Autodesk Inventor part; units mm, degrees
ref_plane "YZ Plane" through (0, 0, 0) normal (1, 0, 0) x (0, 1, 0)
ref_plane "XZ Plane" through (0, 0, 0) normal (0, 1, 0) x (-1, 0, 0)
ref_plane "XY Plane" through (0, 0, 0) normal (0, 0, 1) x (1, 0, 0)
sketch "Sketch1" plane through (0, 0, 0) normal (0, 1, 0) x (-1, 0, 0)
  line L0 (-50, 86.6025) -> (-50, -86.6025)
  line L1 (50, -86.6025) -> (50, 86.6025)
  arc A0 (50, 86.6025) -> (-50, 86.6025) centre (0, 0) ccw
  arc A1 (-50, -86.6025) -> (50, -86.6025) centre (0, 0) ccw
  circle A2 centre (42, -84.8528) radius 1.3
  circle A3 centre (42, -60.6528) radius 1.3
  circle A4 centre (-42, -84.8528) radius 1.3
  circle A5 centre (-42, -60.6528) radius 1.3
  circle A6 centre (42, 84.8528) radius 1.3
  circle A7 centre (42, 60.6528) radius 1.3
  circle A8 centre (-42, 84.8528) radius 1.3
  circle A9 centre (-42, 60.6528) radius 1.3
  circle A10 centre (37.5, -41.0117) radius 5
  circle A11 centre (-37.5, -41.0117) radius 5
  line L2 (10.5, 0) -> (10.5, 43)
  line L3 (10.5, 43) -> (-10.5, 43)
  line L4 (-10.5, 43) -> (-10.5, 0)
  line L5 (10.5, 0) -> (-10.5, 0)
  circle A12 centre (-5.4, -3.5) radius 1.3
  circle A13 centre (5.4, -3.5) radius 1.3
  circle A14 centre (5.4, 46.5) radius 1.3
  circle A15 centre (-5.4, 46.5) radius 1.3
  circle A16 centre (-2.7764, -36.0117) radius 16.406
extrude "Extrusion1" add sketch "Sketch1" against normal blind 3 contours A0 L1 A1 L0 | A16
sketch "Sketch2" plane through (0, 0, 0) normal (0, 1, 0) x (1, 0, 0)
  line L0 (-10.966, 9.168) -> (9.0417, 9.168)
  line L1 (9.0417, 9.168) -> (9.0417, 12.4204)
  line L2 (9.0417, 12.4204) -> (-10.966, 12.4204)
  line L3 (-10.966, 12.4204) -> (-10.966, 9.168)
  line L4 (-10.966, -53.1278) -> (9.0417, -53.1278)
  line L5 (9.0417, -53.1278) -> (9.0417, -56.1278)
  line L6 (9.0417, -56.1278) -> (-10.966, -56.1278)
  line L7 (-10.966, -56.1278) -> (-10.966, -53.1278)
  point P0 (0, 0)
extrude "Extrusion2" cut sketch "Sketch2" against normal blind 3
properties part number "topPlate1"
Check sheet for the modelled part. Datum: model origin and axes. Units: mm. Give positions to 0.01 mm unless a question says otherwise; leave off trailing zeros. Write each loop counter-clockwise with the first axis right and the second up, starting at its lowest first coordinate (ties: lowest second). Pieces come first, ordered by that corner, then holes. Notation, with made-up numbers: (17.25, 61) - (51.25, 61) arc R30 ccw to (51.25, 93) - close; hole circle Ø8 at (40, -37.75). An arc over 180 degrees is marked (long way). Answer as a JSON object with one key per item and string values. Group by question number.
1) Thickness scan on probe 1 along Z at (x, y) = (2, -0.55); probe 2 along Z at (x, y) = (5.4, -1.75); probe 3 along X at (y, z) = (-0.35, -39.5). Record the ranges inside material, lowest first. Write a range as from..to.
2) Release check for a two-part mould opening along X. For faces 1 (the face through (-0.733, -1.479, 99.997)), 2 (the face through (12, -3, 1)), 3 (the face through (41.185, -1.479, -37.632)) record: pulls with the +X half, pulls with the -X half, needs draft (parallel to the pull), parting line crosses it, or undercut.
3) Depth check by flat-ended pin: P1, Ø1, axis at x = -11, y = -2.5, coming from the +Z side; P2, Ø1, axis at x = 17.5, y = -1.5, coming from the -Z side; P3, Ø0.9, axis at x = 2, y = -1, coming from the -Z side. Enter the tip coordinate at first touch or a pass-through.
4) Sectioned sample at A-A (z = 2.5). Record the cut outline in (x, y).
5) Sectioned sample at C-C (y = -1.7). Give the number of separate pieces and of enclosed holes in the cut face, then the cut area to 3 significant figures.
6) Sectioned sample at B-B (x = 37.5). Record the cut outline in (y, z), then the cut area to 3 significant figures.
7) Sectioned sample at D-D (x = -19.5). Record the cut outline in (y, z), then the cut area to 3 significant figures.
Geometry results:
{
 "1": {"probe 1": "z = -99.98..-12.42, -9.17..0, 43..53.13, 56.13..99.98", "probe 2": "z = -99.85..-12.42, -9.17..-4.8, -2.2..0, 43..45.2, 47.8..53.13, 56.13..99.85", "probe 3": "x = -50..-42.27, -32.73..32.73, 42.27..50"},
 "2": {"face 1": "parting line crosses it", "face 2": "needs draft", "face 3": "undercut"},
 "3": {"P1": "stops at z = 99.45", "P2": "stops at z = -98.54", "P3": "stops at z = -99.99"},
 "4": {"outline": "(-50, -3) - (-10.5, -3) - (-10.5, 0) - (-50, 0) - close; (10.5, -3) - (50, -3) - (50, 0) - (10.5, 0) - close"},
 "5": {"separate pieces": "1", "enclosed holes": "17", "area": "17,900 mm^2"},
 "6": {"outline": "(-3, -92.7) - (0, -92.7) - (0, -46.01) - (-3, -46.01) - close; (-3, -36.01) - (0, -36.01) - (0, 92.7) - (-3, 92.7) - close", "area": "526 mm^2"},
 "7": {"outline": "(-3, -98.08) - (0, -98.08) - (0, 98.08) - (-3, 98.08) - close", "area": "588 mm^2"}
}
